```python
from build123d import *

# Parameters (mm, degrees)
EXTRUDE_1_DEPTH     = 4
SKETCH_2_R          = 1
CUT_EXTRUDE_1_DEPTH = 10
SKETCH_3_R          = 1
CUT_EXTRUDE_2_DEPTH = 5


with BuildPart() as part:
    # 草图1 → 凸台-拉伸1 (new body)
    with BuildSketch(Plane.XY):
        with BuildLine():
            Line((2.873991467, 8.252459404), (2.873991467, -7.497540596))
            add(Edge.make_bspline(
                [(2.873991467, -7.497540596), (2.876380091, -7.703382966), (2.699447856, -8.096674523), (2.307764461, -8.248651724), (2.123991437, -8.247540596)],
                knots=[0, 0, 0, 0, 0.528701234, 1, 1, 1, 1], degree=3))
            Line((2.123991437, -8.247540596), (-0.376008504, -8.247540596))
            add(Edge.make_bspline(
                [(-0.376008504, -8.247540596), (-0.778705468, -8.257378213), (-1.13584565, -7.900237207), (-1.126008504, -7.497540596)],
                knots=[0, 0, 0, 0, 1, 1, 1, 1], degree=3))
            Line((-1.126008504, -7.497540596), (-1.126008504, -5.231853607))
            add(Edge.make_bspline(
                [(-1.126008504, -5.231853607), (-1.13659163, -4.751735199), (-1.378371208, -4.02376985), (-2.103997508, -3.523981437), (-2.680544309, -2.960520138), (-2.876380091, -2.341140701), (-2.876008504, -1.924665096)],
                knots=[0, 0, 0, 0, 0.381620227, 0.529034697, 0.676294459, 1, 1, 1, 1], degree=3))
            Line((-2.876008504, -1.924665096), (-2.876008504, 8.252459404))
            Line((-2.876008504, 8.252459404), (-1.776008599, 8.252459404))
            Line((-1.776008599, 8.252459404), (-1.776008599, -1.247540596))
            Line((-1.776008599, -1.247540596), (0.973991401, -1.247540596))
            Line((0.973991401, -1.247540596), (0.973991401, 8.252459404))
            Line((0.973991401, 8.252459404), (2.873991467, 8.252459404))
        make_face()
    extrude(amount=EXTRUDE_1_DEPTH)

    # 草图2 → 切除-拉伸1 (cut)
    with BuildSketch(Plane.ZY.offset(2.876008504)):
        with Locations((2, 5.752459404)):
            Circle(SKETCH_2_R)
    extrude(amount=-CUT_EXTRUDE_1_DEPTH, mode=Mode.SUBTRACT)

    # 草图3 → 切除-拉伸2 (cut)
    with BuildSketch(Plane.XZ.offset(8.247540596)):
        with Locations(Location((0.873991437, 2, 0), (0, 0, 270))):
            Circle(SKETCH_3_R)
    extrude(amount=-CUT_EXTRUDE_2_DEPTH, mode=Mode.SUBTRACT)


solid = part.part
```
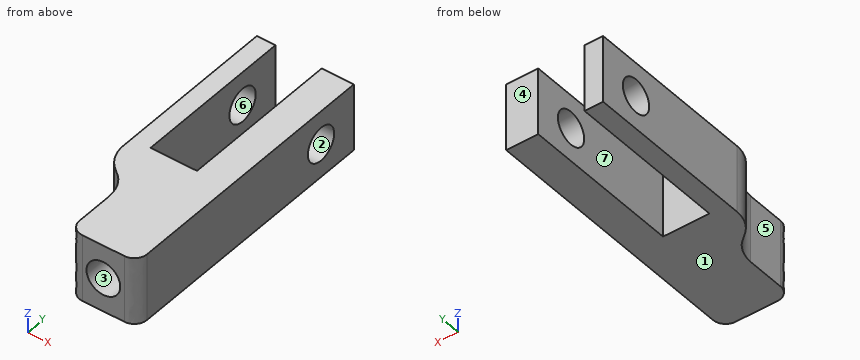
The listing builds one solid part. Answer for the finished solid, in the listing's coordinates (mm). Face numbers are marked on the shaded views. A direction names the side the tool comes from. Give positions to 0.01 mm unless a question says otherwise; leave off trailing zeros. Order: outer loops, then holes, each group sorted by start corner. A loop starts at its lowest first (then second) coordinate and runs counter-clockwise, first axis right, second up. Notation, with made-up numbers: (-7, -9) - (40, -9) arc R16 ccw to (40, 11) - close; hole circle Ø2 at (9, -13.5). An arc over 180 degrees is marked (long way). Use one line per item in the form item = value. Start each with the question number.
(1) The mould has two halves that part along Z. Classify the marked faces 1, 2, 3 and 4: released by +Z, released by -Z, zero draft, split by the parting line, or undercut.
(2) A cutting plane is placed at C-C, the plane y = 6.25. Write down the section's boundary in (x, z).
(3) A cutting plane is placed at A-A, the plane y = 4. Write down the section's boundary in (x, z).
(4) For the marked faces 5, 6 and 7, determine the directions among +Z, -Z, +X, -X, +Y, -Y from which every point of the face is accessible in a straight line to the end or side of a thin tool.
(5) A cutting plane is placed at B-B, the plane z = 2. State how many separate pieces and enclosed holes the cut face has, then the cut area to 3 significant figures.
(6) Consider line 1 (X direction, y = -0.75, z = 0.75); line 2 (Z direction, x = 1.15, y = 5.75); line 3 (Y direction, x = 1.4, z = 2). Determine where each line is inside the solid, lowest interval first. Write a range as from..to.
(7) Flat-ended cylindrical pins translate along their axes: pin 1 Ø1 at (x, z) = (0.5, 2) entering from -Y; pin 2 Ø1.6 at (y, z) = (5.75, 2) entering from -X. Find the tip coordinate at first contact, or state that the pin passes through.
Ans:
q1.face_1 = released by -Z
q1.face_2 = undercut
q1.face_3 = undercut
q1.face_4 = zero draft
q2.outline = (-2.88, 0) - (-1.78, 0) - (-1.78, 1.13) - (-2.88, 1.13) - close; (-2.88, 2.87) - (-1.78, 2.87) - (-1.78, 4) - (-2.88, 4) - close; (0.97, 0) - (2.87, 0) - (2.87, 1.13) - (0.97, 1.13) - close; (0.97, 2.87) - (2.87, 2.87) - (2.87, 4) - (0.97, 4) - close
q3.outline = (-2.88, 0) - (-1.78, 0) - (-1.78, 4) - (-2.88, 4) - close; (0.97, 0) - (2.87, 0) - (2.87, 4) - (0.97, 4) - close
q4.face_5 = +Z, -Z, -X, -Y
q4.face_6 = +X, -X
q4.face_7 = +Z, -Z, +Y
q5.separate_pieces = 3
q5.enclosed_holes = 0
q5.area = 44.3 mm^2
q6.line_1 = -2.88..-1.78, 0.97..2.87
q6.line_2 = 0..1, 3..4
q6.line_3 = -3.25..4.75, 6.75..8.25
q7.pin_1 = -3.25
q7.pin_2 = through
